The model under review builds one solid part; all positions refer to its coordinate system, in mm. A direction names the side the tool comes from. Coordinates: 2 decimals unless noted, no trailing zeros. Write each loop counter-clockwise with the first axis right and the second up, starting at its lowest first coordinate (ties: lowest second). Pieces come first, ordered by that corner, then holes. Notation, with made-up numbers: (-3, 62.25) - (1, 62.25) arc R31 ccw to (1, 101.25) - close; hole circle Ø5 at (6, 83.5). An arc over 180 degrees is marked (long way). Return JSON: item names as keys, results as strings. Group by question number.
(1) We need section D-D on x = 22. Give the number of separate pieces and of enclosed holes in the cut face, then the cut area to 3 significant figures.
(2) We need section A-A on y = 0. State the section outline as (x, z) points (3 decimals).
(3) To check wall thickness, follow L1, parallel to Y at x = 15.75, z = -27.5; L2, parallel to Y at x = 14, z = -28.5; L3, parallel to Z at x = 24.25, y = 35.5. State the ranges of each line that lie inside material, in increasing order. Write a range as from..to.
(4) Tool access review of faces 1 (the face through (19.14, 48.11, -1.38)), 2 (the face through (12.7, -13, 11)): name each direction out of +Z, -Z, +X, -X, +Y, -Y from which nothing blocks a thin tool from reaching the whole face with its end or side.
(5) Draft analysis for pull direction Z (two halves, no side actions). For faces 3 (the face through (6.439, -3.441, -15.497)), 4 (the face through (0, 0, 7)), 5 (the face through (19.14, -17.24, -44.54)), state which applies: released by +Z, released by -Z, zero draft, split by the parting line, or undercut.
(6) For pin 1 Ø1 at (x, z) = (9.5, 0) entering from -Y (3 decimals); pin 2 Ø1 at (y, z) = (15.5, 43) entering from +X; pin 3 Ø14.5 at (y, z) = (33.91, 24.63) entering from -X; pin 4 Ø6 at (x, z) = (13.5, 5) entering from +Y, all flat-tipped, find the tip position at first contact; note any pin that passes through.
(7) We need section B-B on z = 28.5. State the section outline as (x, y) points.
Autodesk Inventor part; units mm, degrees
ref_plane "YZ Plane" through (0, 0, 0) normal (1, 0, 0) x (0, 1, 0)
ref_plane "XZ Plane" through (0, 0, 0) normal (0, 1, 0) x (-1, 0, 0)
ref_plane "XY Plane" through (0, 0, 0) normal (0, 0, 1) x (1, 0, 0)
sketch "Sketch1" plane through (0, 0, 0) normal (0, 0, 1) x (1, 0, 0)
  line L0 (0, 0) -> (0, 15.875)
  line L1 (0, 15.875) -> (12.7, 15.875)
  line L2 (12.7, 15.875) -> (12.7, 53.975)
  line L3 (12.7, 53.975) -> (25.4, 53.975)
  line L4 (25.4, 53.975) -> (25.4, 0)
  line L5 (25.4, 0) -> (0, 0)
  dimension "d0" = 15.875
  dimension "d1" = 12.7
  dimension "d2" = 38.1
  dimension "d3" = 12.7
revolve "Revolution1" add sketch "Sketch1" angle 360 about axis through (25.4, 0, 0) along (-1, 0, 0)
sketch "Sketch2" plane through (0, 0, 0) normal (-1, 0, 0) x (0, 0, 1)
  point P0 (0, 0)
  point P1 (0, 0)
hole "Hole1" at (0, 0, 0) direction (1, 0, 0) diameter 12.7 end through all
sketch "Sketch3" plane through (12.7, 0, 0) normal (-1, 0, 0) x (0, 0, 1)
  circle A0 centre (0, 0) radius 41.91 construction
  point P0 (0, 83.82)
  point P1 (0, 41.91)
  point P2 (-24.6341, 33.9059)
  point P3 (-39.8588, 12.9509)
  point P4 (-39.8588, -12.9509)
  point P5 (-24.6341, -33.9059)
  point P6 (0, -41.91)
  point P7 (24.6341, -33.9059)
  point P8 (39.8588, -12.9509)
  point P9 (39.8588, 12.9509)
  point P10 (24.6341, 33.9059)
  dimension "d13" = 83.82
  dimension "d16" = 360
hole "Hole2" at (12.7, 83.82, 0) at (12.7, 41.91, 0) at (12.7, 33.9059, -24.6341) at (12.7, 12.9509, -39.8588) at (12.7, -12.9509, -39.8588) at (12.7, -33.9059, -24.6341) at (12.7, -41.91, 0) at (12.7, -33.9059, 24.6341) at (12.7, -12.9509, 39.8588) at (12.7, 12.9509, 39.8588) at (12.7, 33.9059, 24.6341) direction (1, 0, 0) diameter 12.7 end through all
sketch "Sketch4" plane through (0, 0, 0) normal (-1, 0, 0) x (0, 0, 1)
  circle A0 centre (0, 0) radius 6.35
  line L0 (0, 0) -> (0, 10.0164) construction
  line L1 (0, 6.35) -> (0.6342, 6.3182)
  line L2 (0, 6.35) -> (-0.6358, 6.3181)
  line L3 (-0.6358, 6.3181) -> (-0.6994, 7.5865)
  line L4 (-0.6994, 7.5865) -> (0.5706, 7.5865)
  line L5 (0.5706, 7.5865) -> (0.6342, 6.3182)
  dimension "d27" = 0.635
  dimension "d28" = 1.27
  dimension "d29" = 1.27
extrude "Extrusion1" cut sketch "Sketch4" against normal up to next contours A0 L3 L4 L5
properties part number "CircularPattern"
Ans:
{
 "1": {"separate pieces": "1", "enclosed holes": "11", "area": "7,760 mm²"},
 "2": {"outline": "(0, -15.875) - (12.7, -15.875) - (12.7, -53.975) - (25.4, -53.975) - (25.4, -6.35) - (0, -6.35) - close; (0, 6.35) - (25.4, 6.35) - (25.4, 53.975) - (12.7, 53.975) - (12.7, 15.875) - (0, 15.875) - close"},
 "3": {"L1": "-46.44..-39.57, -28.24..28.24, 39.57..46.44", "L2": "-45.84..-38.94, -28.87..28.87, 38.94..45.84", "L3": "-40.66..-30.78, -18.49..18.49, 30.78..40.66"},
 "4": {"face 1": "+X, -X", "face 2": "-X"},
 "5": {"face 3": "split by the parting line", "face 4": "zero draft", "face 5": "undercut"},
 "6": {"pin 1": "y = -15.875", "pin 2": "through", "pin 3": "x = 12.7", "pin 4": "y = 53.94"},
 "7": {"outline": "(12.7, -45.84) - (25.4, -45.84) - (25.4, -38.94) - (12.7, -38.94) - close; (12.7, -28.87) - (25.4, -28.87) - (25.4, 28.87) - (12.7, 28.87) - close; (12.7, 38.94) - (25.4, 38.94) - (25.4, 45.84) - (12.7, 45.84) - close"}
}
